Input: dimensioned drawing with shaded views. Units: mm. Origin: part minimum x, y, z. A direction names the side the tool comes from. Give positions to 0.01 mm unless a question says otherwise; leave off trailing zeros. Write each loop counter-clockwise with the first axis right and the second up, starting at its lowest first coordinate (ties: lowest second). Pieces come first, ordered by that corner, then holes.
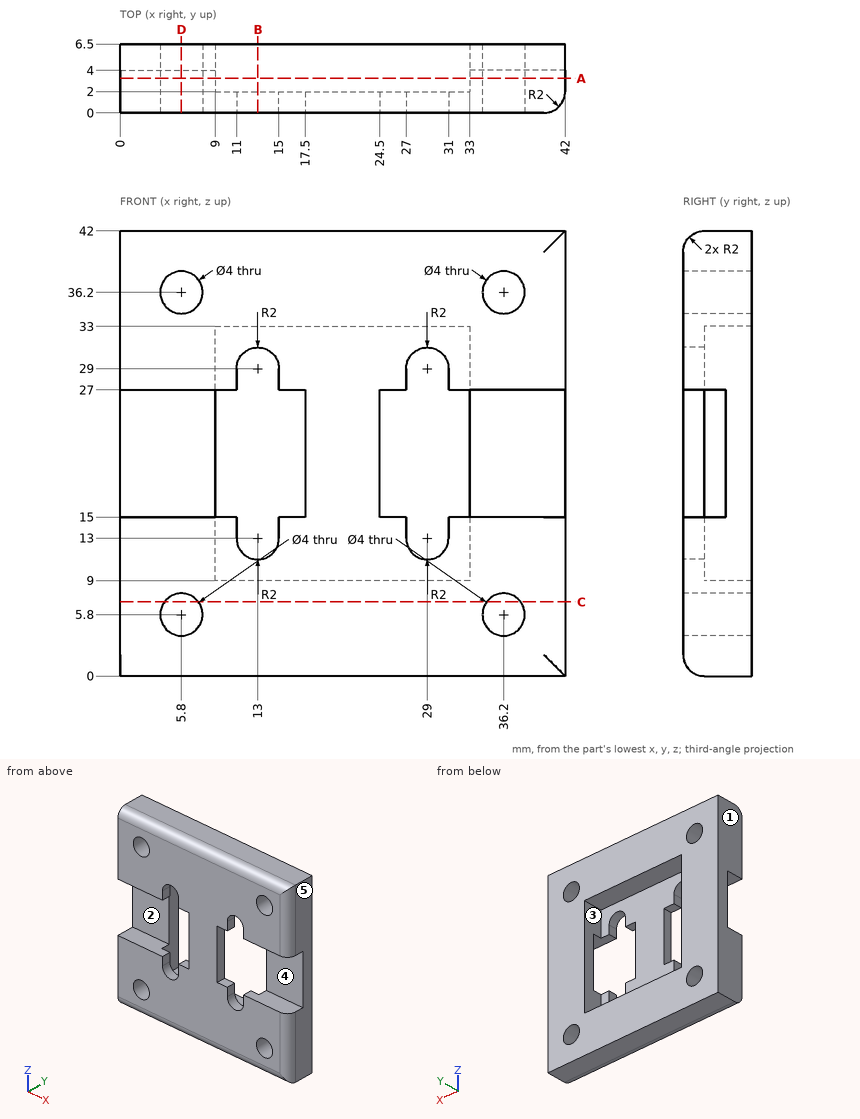
Item 1: Reachability of the marked faces 1, 2 and 3 from +Z, -Z, +X, -X, +Y, -Y: full face, straight path, thin tool, end or side. Return the list, or none.
Found:
face 1: +Z, -Z, -X, +Y, -Y
face 2: +X, -X, -Y
face 3: +Y
Item 2: Section D-D, the plane x = 5.8. Return the cut outline in (y, z).
Found:
outline: (0, 2) arc R2 ccw to (2, 0) - (6.5, 0) - (6.5, 3.8) - (0, 3.8) - close; (0, 7.8) - (6.5, 7.8) - (6.5, 34.2) - (0, 34.2) - (0, 27) - (4, 27) - (4, 15) - (0, 15) - close; (0, 38.2) - (6.5, 38.2) - (6.5, 42) - (2, 42) arc R2 ccw to (0, 40) - close
Item 3: Pull-direction query (Z, two-part tool) for the marked faces 4 and 5; classes: +Z half, -Z half, draft (parallel to the pull), parting line (faces both ways), or undercut.
Found:
face 4: undercut
face 5: draft
Item 4: Section A-A, the plane y = 3.25. Return the cut outline in (x, z), plus the area to 3 significant figures.
Found:
outline: (0, 0) - (42, 0) - (42, 15) - (33, 15) - (33, 9) - (9, 9) - (9, 15) - (0, 15) - close; (0, 27) - (9, 27) - (9, 33) - (33, 33) - (33, 27) - (42, 27) - (42, 42) - (0, 42) - close; hole circle Ø4 at (5.8, 5.8); hole circle Ø4 at (5.8, 36.2); hole circle Ø4 at (36.2, 5.8); hole circle Ø4 at (36.2, 36.2)
area: 922 mm2
Item 5: Section B-B, the plane x = 13. Return the cut outline in (y, z), plus the area to 3 significant figures.
Found:
outline: (0, 2) arc R2 ccw to (2, 0) - (6.5, 0) - (6.5, 9) - (2, 9) - (2, 11) - (0, 11) - close; (0, 31) - (2, 31) - (2, 33) - (6.5, 33) - (6.5, 42) - (2, 42) arc R2 ccw to (0, 40) - close
area: 123 mm2
Item 6: Section C-C, the plane z = 7. Return the cut outline in (x, y).
Found:
outline: (0, 0) - (4.2, 0) - (4.2, 6.5) - (0, 6.5) - close; (7.4, 0) - (34.6, 0) - (34.6, 6.5) - (7.4, 6.5) - close; (37.8, 0) - (40, 0) arc R2 ccw to (42, 2) - (42, 6.5) - (37.8, 6.5) - close
Item 7: Pin query (flat end, axial travel): pin 1 Ø0.6 at (x, y) = (16, 1) entering from -Z; pin 2 Ø1.6 at (y, z) = (0.5, 14.5) entering from +X; pin 3 Ø1.5 at (y, z) = (1, 18.5) entering from -X; pin 4 Ø3.5 at (x, z) = (5.8, 5.8) entering from +Y. Return the tip coordinate at first contact, or that it passes through.
Found:
pin 1: stops at z = 0.13
pin 2: stops at x = 41.87
pin 3: stops at x = 17.5
pin 4: passes through
Item 8: Line query: L1, parallel to Z at x = 6, y = 2.5; L2, parallel to X at y = 4.5, z = 36.2; L3, parallel to Z at x = 29, y = 3.5. Output: solid intervals per line, ascending.
Found:
L1: z = 0 to 3.81, 7.79 to 15, 27 to 34.21, 38.19 to 42
L2: x = 0 to 3.8, 7.8 to 34.2, 38.2 to 42
L3: z = 0 to 9, 33 to 42
